Input: dimensioned drawing with shaded views. Units: mm. Origin: part minimum x, y, z. A direction names the side the tool comes from. Round coordinates to 2 decimals unless told otherwise and drop trailing zeros. Loops run counter-clockwise (first coordinate to the right, second up) from the corner with the lowest first, then second, coordinate; pieces in that order, holes last.
1) Section D-D, the plane z = 1.25. Return loops of the section in (x, y).
2) Section C-C, the plane y = 4.75. Return loops of the section in (x, z), and give its area (3 significant figures).
3) Section B-B, the plane x = 6.75. Return loops of the section in (y, z), and give its area (3 significant figures).
4) Draft query along Y for the marked faces 1, 2, 3 and 4. Return one class per face: pulls with the +Y half, pulls with the -Y half, needs draft (parallel to the pull), parting line crosses it, or undercut.
5) First-contact query: pin 1 (0.9 mm diameter, centred on x = 7, z = 1, fed in from +Y); pin 2 (3 mm diameter, centred on x = 4.5, y = 5.5, fed in from +Z); pin 3 (1.5 mm diameter, centred on y = 5, z = 3, fed in from +X). Flat tips, straight axial feed; report the tip coordinate or a pass-through.
6) Section A-A, the plane z = 4.25. Return loops of the section in (x, y), and give its area (3 significant figures).
7) Access query for the marked faces 5, 6 and 7. Directions: +Z, -Z, +X, -X, +Y, -Y. A direction counts if a zero-diameter tool reaches every point of the face in a straight line with its end or side. Return the directions, or none.
8) Ray query, line 1 along Z through (x, y) = (10.5, 2.5); line 2 along Y through (x, z) = (8.25, 0.75); line 3 along X through (y, z) = (7.75, 3). Return the intervals inside material, ascending.
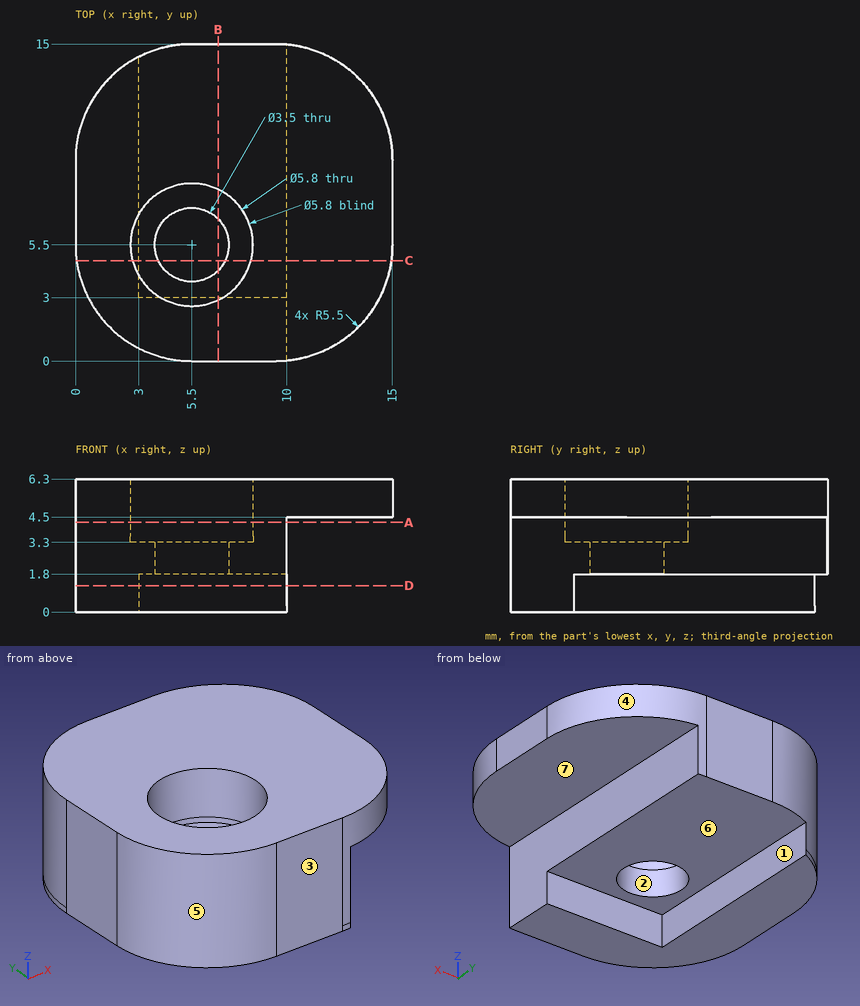
Final values:
1. outline: (0, 5.5) arc R5.5 ccw to (5.5, 0) - (9.5, 0) arc R5.5 ccw to (10, 0.02) - (10, 3) - (3, 3) - (3, 14.4) arc R5.5 ccw to (0, 9.5) - close
2. outline: (0.05, 0) - (3, 0) - (3, 1.8) - (3.92, 1.8) - (3.92, 3.3) - (2.7, 3.3) - (2.7, 6.3) - (0.05, 6.3) - close; (7.08, 1.8) - (10, 1.8) - (10, 4.5) - (14.95, 4.5) - (14.95, 6.3) - (8.3, 6.3) - (8.3, 3.3) - (7.08, 3.3) - close
2. area: 37.4 mm2
3. outline: (0, 0) - (3, 0) - (3, 1.8) - (4.28, 1.8) - (4.28, 3.3) - (2.88, 3.3) - (2.88, 6.3) - (0, 6.3) - close; (6.72, 1.8) - (15, 1.8) - (15, 6.3) - (8.12, 6.3) - (8.12, 3.3) - (6.72, 3.3) - close
3. area: 53.5 mm2
4. face 1: needs draft
4. face 2: undercut
4. face 3: pulls with the -Y half
4. face 4: pulls with the +Y half
5. pin 1: stops at y = 3
5. pin 2: stops at z = 3.3
5. pin 3: stops at x = 10
6. outline: (0, 5.5) arc R5.5 ccw to (5.5, 0) - (9.5, 0) arc R5.5 ccw to (10, 0.02) - (10, 14.98) arc R5.5 ccw to (9.5, 15) - (5.5, 15) arc R5.5 ccw to (0, 9.5) - close; hole circle Ø5.8 at (5.5, 5.5)
6. area: 111 mm2
7. face 5: +Z, -Z, -X, -Y
7. face 6: -Z, +X, +Y
7. face 7: -Z, +X, +Y, -Y
8. line 1: z = 4.5 to 6.3
8. line 2: y = 0 to 3
8. line 3: x = 0 to 10
